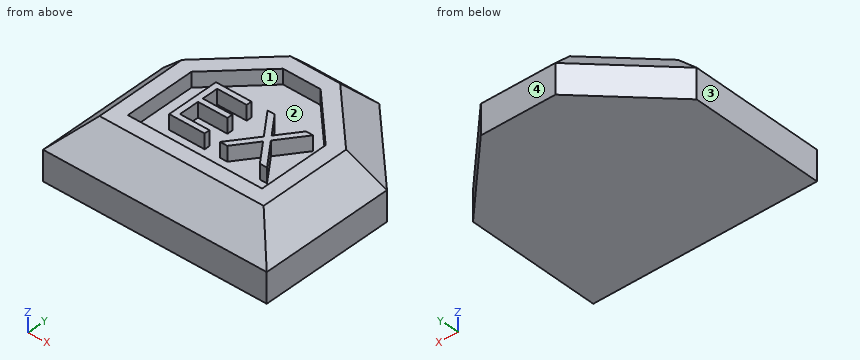
```python
from build123d import *

# Parameters (mm, degrees)
EXTRUDE_1_DEPTH     = 4
CHAMFER_1_SIZE      = 2
CUT_EXTRUDE_1_DEPTH = 1
EXTRUDE_2_DEPTH     = 1


with BuildPart() as part:
    # 草图1 → 凸台-拉伸1 (new body)
    with BuildSketch(Plane.XY):
        Polygon((-7.5, 2), (-2.5, 7), (2.5, 7), (7.5, 2), (7.5, -7), (-7.5, -7), align=None)
    extrude(amount=EXTRUDE_1_DEPTH)

    # 倒角1
    chamfer_1_edges = [part.edges().sort_by_distance(p)[0] for p in [
        (7.5, -2.5, 4),
        (5, 4.5, 4),
        (0, 7, 4),
        (-5, 4.5, 4),
        (-7.5, -2.5, 4),
        (0, -7, 4),
    ]]
    chamfer(chamfer_1_edges, length=CHAMFER_1_SIZE)

    # 草图2 → 切除-拉伸1 (cut)
    with BuildSketch(Plane.XY.offset(4)):
        Polygon((-4.5, -4), (4.5, -4), (4.5, 0.757359313), (1.257359313, 4), (-1.257359313, 4), (-4.5, 0.757359313), align=None)
    extrude(amount=-CUT_EXTRUDE_1_DEPTH, mode=Mode.SUBTRACT)

    # 草图3 → 凸台-拉伸2 (add)
    with BuildSketch(Plane.XY.offset(3)):
        Polygon((-3.018784833, 0.942914113), (-0.640579705, 0.942914113), (-0.640579705, 0.583939754), (-2.614938679, 0.583939754), (-2.614938679, -0.492983323), (-0.640579705, -0.492983323), (-0.640579705, -0.851957682), (-2.614938679, -0.851957682), (-2.614938679, -2.198111528), (-0.640579705, -2.198111528), (-0.640579705, -2.557085887), (-3.018784833, -2.557085887), align=None)
        Polygon((0.440830551, 0.942914113), (0.920397859, 0.942914113), (1.966471577, -0.45652499), (3.012545295, 0.942914113), (3.492112603, 0.942914113), (2.206255231, -0.77693765), (3.536984397, -2.557085887), (3.05741709, -2.557085887), (1.966471577, -1.098051432), (0.875526064, -2.557085887), (0.395958756, -2.557085887), (1.726687923, -0.77693765), align=None)
    extrude(amount=EXTRUDE_2_DEPTH)


solid = part.part
```
Geometry: final body of the model. Coordinates: model frame, mm. Face numbers are marked on the shaded views. Coordinates: 2 decimals unless noted, no trailing zeros. Order: outer loops, then holes, each group sorted by start corner. A loop starts at its lowest first (then second) coordinate and runs counter-clockwise, first axis right, second up. Notation, with made-up numbers: (68, 6.25) - (93, 6.25) arc R15 ccw to (93, 23.25) - close; hole circle Ø1 at (59, 32). An arc over 180 degrees is marked (long way). Return JSON: item names as keys, results as strings. Group by question number.
1. Material intervals for line 1 along Y through (x, z) = (-7, 0.2); line 2 along Z through (x, y) = (2, 2); line 3 along Y through (x, z) = (4, 1.75), sorted ascending. Write a range as [from, to].
2. Cut plane C-C (y = 3.25). Output: boundary loops of the cut face in (x, z), plus the area to 3 significant figures.
3. Pin query (flat end, axial travel): pin 1 (0.5 mm diameter, centred on y = -0.5, z = 3.5, fed in from +X); pin 2 (1.1 mm diameter, centred on x = 0.5, z = 3.5, fed in from -Y); pin 3 (0.5 mm diameter, centred on x = 0.5, z = 3.5, fed in from -Y). Return the tip coordinate at first contact, or that it passes through.
4. Cut plane D-D (z = 3.55). Count the separate pieces of the cut face and the enclosed holes in it, plus the area to 3 significant figures.
5. Pull-direction query (Y, two-part tool) for the marked faces 1, 2, 3 and 4; classes: pulls with the +Y half, pulls with the -Y half, needs draft (parallel to the pull), parting line crosses it, or undercut.
6. Cut plane A-A (x = -1). Output: boundary loops of the cut face in (y, z), plus the area to 3 significant figures.
7. Cut plane B-B (z = 0.5). Output: boundary loops of the cut face in (x, y).
Resolved:
{
 "1": {"line 1": "y = [-7, 2.5]", "line 2": "z = [0, 3]", "line 3": "y = [-7, 5.5]"},
 "2": {"outline": "(-6.25, 0) - (6.25, 0) - (6.25, 2) - (3.42, 4) - (2.01, 4) - (2.01, 3) - (-2.01, 3) - (-2.01, 4) - (-3.42, 4) - (-6.25, 2) - close", "area": "40.3 mm²"},
 "3": {"pin 1": "stops at x = 6.25", "pin 2": "stops at y = -6.05", "pin 3": "stops at y = -5.75"},
 "4": {"separate pieces": "3", "enclosed holes": "1", "area": "58.2 mm²"},
 "5": {"face 1": "undercut", "face 2": "undercut", "face 3": "needs draft", "face 4": "pulls with the +Y half"},
 "6": {"outline": "(-7, 0) - (7, 0) - (7, 2) - (5, 4) - (4, 4) - (4, 3) - (0.94, 3) - (0.94, 4) - (0.58, 4) - (0.58, 3) - (-0.49, 3) - (-0.49, 4) - (-0.85, 4) - (-0.85, 3) - (-2.2, 3) - (-2.2, 4) - (-2.56, 4) - (-2.56, 3) - (-4, 3) - (-4, 4) - (-5, 4) - (-7, 2) - close", "area": "45.1 mm²"},
 "7": {"outline": "(-7.5, -7) - (7.5, -7) - (7.5, 2) - (2.5, 7) - (-2.5, 7) - (-7.5, 2) - close"}
}
